Autodesk Inventor part; units mm, degrees
ref_plane "YZ Plane" through (0, 0, 0) normal (1, 0, 0) x (0, 1, 0)
ref_plane "XZ Plane" through (0, 0, 0) normal (0, 1, 0) x (-1, 0, 0)
ref_plane "XY Plane" through (0, 0, 0) normal (0, 0, 1) x (1, 0, 0)
sketch "Sketch1" plane through (0, 0, 0) normal (0, 1, 0) x (-1, 0, 0)
  line L0 (11.25, 9.4) -> (-11.25, 9.4)
  line L1 (-11.25, 9.4) -> (-11.25, -9.4)
  line L2 (-11.25, -9.4) -> (11.25, -9.4)
  line L3 (11.25, -9.4) -> (11.25, 9.4)
  line L4 (11.25, 9.4) -> (-11.25, -9.4) construction
  line L5 (-11.25, 9.4) -> (11.25, -9.4) construction
  point P0 (0, 0)
  dimension "d0" = 22.5
  dimension "d1" = 18.8
extrude "Extrusion1" add sketch "Sketch1" along normal blind 37
sketch "Sketch2" plane through (-11.25, 0, 9.4) normal (0, 0, 1) x (1, 0, 0)
  circle A0 centre (11.25, 11.2) radius 2.7
  line L0 (0, 0) -> (22.5, 0)
  line L1 (11.25, 0) -> (11.25, 37) construction
  line L2 (0, 37) -> (22.5, 37)
  dimension "d4" = 5.4
  dimension "d5" = 11.2
extrude "Extrusion2" add sketch "Sketch2" along normal blind 9.5
sketch "Sketch3" plane through (0, 11.2, 18.9) normal (0, 0, 1) x (1, 0, 0)
  circle A0 centre (0, 0) radius 2.7
  line L0 (-2.0125, 1.8) -> (2.0125, 1.8)
  line L1 (-2.0125, -1.8) -> (2.0125, -1.8)
  point P0 (0, -11.2)
  dimension "d8" = 3.6
extrude "Extrusion3" cut sketch "Sketch3" against normal blind 7.9 contours L0 A0 | A0 L1
mirror "Mirror1" about plane through (0, 0, 0) normal (0, 0, 1) of "Extrusion2", "Extrusion3"
sketch "Sketch4" plane through (0, 0, 0) normal (0, -1, 0) x (1, 0, 0)
  line L0 (-2.5, -4.4) -> (2.5, -4.4)
  line L1 (2.5, -4.4) -> (2.5, -1.4)
  line L2 (2.5, -1.4) -> (-2.5, -1.4)
  line L3 (-2.5, -1.4) -> (-2.5, -4.4)
  line L4 (-2.5, -4.4) -> (2.5, -1.4) construction
  line L5 (2.5, -4.4) -> (-2.5, -1.4) construction
  line L6 (-11.25, 9.4) -> (11.25, 9.4) construction
  line L7 (0, -26.46) -> (0, 26.46) construction
  point P0 (0, -2.9)
  point P1 (0, -2.9)
  dimension "d11" = 5
  dimension "d12" = 3
  dimension "d22" = 10.8
extrude "Extrusion4" add sketch "Sketch4" along normal blind 5
sketch "Sketch5" plane through (2.5, 0, -4.4) normal (0, 0, -1) x (-1, 0, 0)
  circle A0 centre (2.5, -2.6) radius 1.4
  line L0 (5, -5) -> (0, -5) construction
  line L1 (2.5, 0) -> (2.5, -5) construction
  dimension "d15" = 2.8
  dimension "d16" = 2.4
extrude "Extrusion5" cut sketch "Sketch5" against normal up to next
sketch "Sketch6" plane through (0, 37, 0) normal (0, 1, 0) x (1, 0, 0)
  line L0 (11.25, 9.4) -> (-11.25, 9.4)
  line L1 (11.25, -9.4) -> (11.25, 9.4)
  line L2 (-11.25, 9.4) -> (11.25, 9.4)
  line L3 (11.25, 9.4) -> (11.25, -5.7)
  line L4 (11.25, -5.7) -> (-11.25, -5.7)
  line L5 (-11.25, -5.7) -> (-11.25, 9.4)
  line L6 (-11.25, -9.4) -> (11.25, -9.4)
  circle A0 centre (0, 1.85) radius 11.25
  line L7 (-11.25, 9.4) -> (-11.25, -9.4)
  line L8 (11.25, -9.4) -> (11.25, 9.4)
  point P0 (0, 0)
  point P1 (-8.3403, 9.4)
  point P2 (-8.3403, -5.7)
  point P3 (8.3403, -5.7)
  point P4 (8.3403, 9.4)
  dimension "d19" = 3.7
  dimension "d23" = 15.1
  dimension "d24" = 7.55
extrude "Extrusion6" add sketch "Sketch6" along normal blind 27.2 contours A0 L4 L0
sketch "Sketch7" plane through (-11.25, 0, 9.4) normal (0, 0, 1) x (1, 0, 0)
  circle A0 centre (2.5, 31.1) radius 1.4
  line L0 (0, 0) -> (22.5, 0)
  line L1 (0, 37) -> (22.5, 37) construction
  circle A1 centre (20, 31.1) radius 1.4
  line L2 (0, 0) -> (0, 37)
  point P0 (11.25, 0)
  dimension "d25" = 2.8
  dimension "d26" = 31.1
  dimension "d29" = 17.5
  dimension "d34" = 22.5
  dimension "d35" = 2.5
extrude "Extrusion7" cut sketch "Sketch7" against normal blind 4
fillet "Fillet1" radius 3 2 edges at (11.25, 0, 0) (-11.25, 0, 0)
equation "\"d24\" = 0.5 * d23"
equation "\"d35\" = -0.5 * d29 + 0.5 * d34"
properties part number "motor3"
Design review of the part built by this model. Coordinates are the model's own, in mm. A direction names the side the tool comes from. Give positions to 0.01 mm unless a question says otherwise; leave off trailing zeros. Write each loop counter-clockwise with the first axis right and the second up, starting at its lowest first coordinate (ties: lowest second). Pieces come first, ordered by that corner, then holes.
(1) Add section A-A (y = -2.6). Give the boundary of the cut face in (x, z), and give its area (3 significant figures).
Checked values:
outline: (-2.5, -4.4) - (-1.4, -4.4) - (-1.4, -1.4) - (-2.5, -1.4) - close; (1.4, -4.4) - (2.5, -4.4) - (2.5, -1.4) - (1.4, -1.4) - close
area: 6.60 mm2
(2) Add section C-C (z = 7). Give the boundary of the cut face in (x, y), and give its area (3 significant figures).
Checked values:
outline: (-11.25, 3) arc R3 ccw to (-8.25, 0) - (8.25, 0) arc R3 ccw to (11.25, 3) - (11.25, 37) - (-11.25, 37) - close; hole circle Ø2.8 at (-8.75, 31.1); hole circle Ø2.8 at (8.75, 31.1)
area: 816 mm2
(3) Mouldability with a two-part tool opening along X and no side actions: class faces 5 (the face through (0, 11, -18.9)), 6 (the face through (8.57, 32.49, 7.43)), 7 (the face through (-11.25, 20, 0)), 8 (the face through (-0.75, -1.42, -2.92)) as +X half, -X half, draft (parallel to the pull), parting line (faces both ways), or undercut.
Checked values:
face 5: draft
face 6: undercut
face 7: -X half
face 8: undercut
(4) Clearance check with flat-ended pins moving along their axes: pin 1 Ø0.9 at (y, z) = (-3.5, -3.5) entering from -X; pin 2 Ø8 at (x, y) = (8, 42.5) entering from +Z; pin 3 Ø0.5 at (x, y) = (0, 13.5) entering from +Z; pin 4 Ø3.5 at (x, z) = (3, 6) entering from +Y. State where each tip first meets the part, or that it passes through.
Checked values:
pin 1: stops at x = -2.5
pin 2: stops at z = 5.7
pin 3: stops at z = 11
pin 4: stops at y = 64.2
(5) Tool access review of faces 1 (the face through (-11.25, 50.41, -1.73)), 2 (the face through (1, -1, -4.4)), 3 (the face through (2.494, 12.234, 13.028)), 4 (the face through (0, 9.4, 15)): name each direction out of +Z, -Z, +X, -X, +Y, -Y from which nothing blocks a thin tool from reaching the whole face with its end or side.
Checked values:
face 1: -X, +Y
face 2: -Z, +X, -X, -Y
face 3: +Z
face 4: +Z, +X, -X, -Y
(6) Add section D-D (y = 11.2). Give the boundary of the cut face in (x, z).
Checked values:
outline: (-11.25, -9.4) - (-2.7, -9.4) - (-2.7, -18.9) - (2.7, -18.9) - (2.7, -9.4) - (11.25, -9.4) - (11.25, 9.4) - (2.7, 9.4) - (2.7, 18.9) - (-2.7, 18.9) - (-2.7, 9.4) - (-11.25, 9.4) - close
(7) Wall thickness on line 1 along X through (y, z) = (31, 6); line 2 along Y through (x, z) = (-1.25, 15.5); line 3 along Z through (x, y) = (-1, 14): over which ranges is each line inside the solid? List them lowest first.
Checked values:
line 1: x = -11.25 to -10.15, -7.35 to 7.35, 10.15 to 11.25
line 2: y = 9.4 to 13
line 3: z = -9.4 to 9.4
